```python
from build123d import *

# Parameters (mm, degrees)
F2_W     = 20
F2_H     = 20
F3_DEPTH = 140
F4_R     = 3
F5_T     = -2
F7_DEPTH = 20.001
F9_DEPTH = 25


with BuildPart() as f3:
    # F2 (on Front) → F3 (new body, symmetric)
    with BuildSketch(Plane.XZ):
        Rectangle(F2_W, F2_H)
    extrude(amount=F3_DEPTH, both=True)

    # F4
    f4_edges = [f3.edges().sort_by_distance(p)[0] for p in [
        (10, 0, 10),
        (-10, 0, 10),
        (10, 0, -10),
        (-10, 0, -10),
    ]]
    fillet(f4_edges, radius=F4_R)

    # F5
    f5_openings = [f3.faces().sort_by_distance(p)[0] for p in [
        (0, -140, 0),
        (0, 140, 0),
    ]]
    offset(amount=F5_T, openings=f5_openings)

    # F6 (on face) → F7 (cut, through all)
    with BuildSketch(Plane(origin=(-10, 0, 0), x_dir=(0, -1, 0), z_dir=(-1, 0, 0))):
        Polygon((-120, 10), (-140, 10), (-140, -10), align=None)
    extrude(amount=-F7_DEPTH, mode=Mode.SUBTRACT)

    # F8 (on face) → F9 (cut)
    with BuildSketch(Plane(origin=(0, 0, -10), x_dir=(1, 0, 0), z_dir=(0, 0, -1))):
        Polygon((10, 140), (-10, 140), (-10, 120), align=None)
    extrude(amount=-F9_DEPTH, mode=Mode.SUBTRACT)


solid = f3.part
```
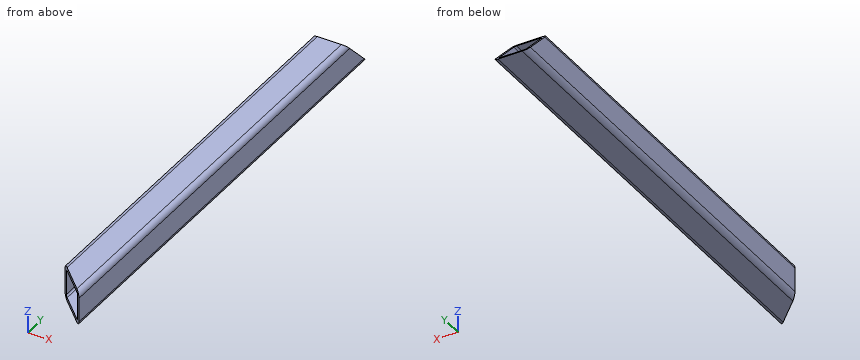
Design review of the part built by this model. Coordinates are the model's own, in mm. Give positions to 0.01 mm unless a question says otherwise; leave off trailing zeros. Write each loop counter-clockwise with the first axis right and the second up, starting at its lowest first coordinate (ties: lowest second). Pieces come first, ordered by that corner, then holes.
(1) Add section A-A (z = -1.75). Give the boundary of the cut face in (x, y).
Checked values:
outline: (-10, -120) - (-8, -122) - (-8, 131.75) - (-10, 131.75) - close; (8, -138) - (10, -140) - (10, 131.75) - (8, 131.75) - close
(2) Clearance check with a flat-ended pin moving along its axis: pin 1 Ø12 at (x, z) = (-4, -6) entering from -Y. State where the tip first meets the part, or that it passes through.
Checked values:
pin 1: stops at y = -131.66
(3) Add section C-C (y = -52). Give the boundary of the cut face in (x, z).
Checked values:
outline: (-10, -7) arc R3 ccw to (-7, -10) - (7, -10) arc R3 ccw to (10, -7) - (10, 7) arc R3 ccw to (7, 10) - (-7, 10) arc R3 ccw to (-10, 7) - close; hole (-8, -7) arc R1 ccw to (-7, -8) - (7, -8) arc R1 ccw to (8, -7) - (8, 7) arc R1 ccw to (7, 8) - (-7, 8) arc R1 ccw to (-8, 7) - close
(4) Add section B-B (x = 0.25). Give the boundary of the cut face in (y, z).
Checked values:
outline: (-130.25, -10) - (140, -10) - (138, -8) - (-130.25, -8) - close; (-130.25, 8) - (122, 8) - (120, 10) - (-130.25, 10) - close
(5) Wall thickness on line 1 along X through (y, z) = (53, 2.5); line 2 along X through (y, z) = (-124, -3.75): over which ranges is each line inside the solid? List them lowest first.
Checked values:
line 1: x = -10 to -8, 8 to 10
line 2: x = 8 to 10
